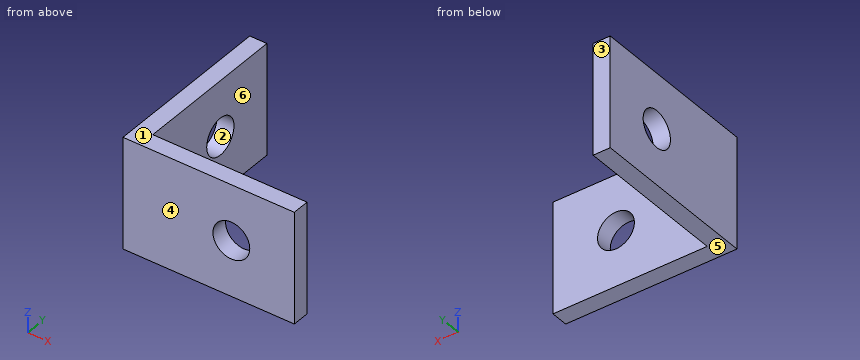
from build123d import *

# Parameters (mm, degrees)
BOSS_EXTRUDE1_DEPTH = 13
SKETCH2_R           = 2.15
CUT_EXTRUDE1_DEPTH  = 21
SKETCH3_R           = 2.15
CUT_EXTRUDE2_DEPTH  = 21


with BuildPart() as part:
    # Sketch1 → Boss-Extrude1 (new body)
    with BuildSketch(Plane.XY):
        Polygon((0, 20), (0, 0), (20, 0), (20, 2), (2, 2), (2, 20), align=None)
    extrude(amount=BOSS_EXTRUDE1_DEPTH)

    # Sketch2 → Cut-Extrude1 (cut, through all)
    with BuildSketch(Plane.ZY):
        with Locations((6.5, 12.65)):
            Circle(SKETCH2_R)
    extrude(amount=-CUT_EXTRUDE1_DEPTH, mode=Mode.SUBTRACT)

    # Sketch3 → Cut-Extrude2 (cut, through all)
    with BuildSketch(Plane.XZ):
        with Locations((12.65, 6.5)):
            Circle(SKETCH3_R)
    extrude(amount=-CUT_EXTRUDE2_DEPTH, mode=Mode.SUBTRACT)


solid = part.part
The model under review builds one solid part; all positions refer to its coordinate system, in mm. Face numbers are marked on the shaded views. A direction names the side the tool comes from. Coordinates: 2 decimals unless noted, no trailing zeros. Write each loop counter-clockwise with the first axis right and the second up, starting at its lowest first coordinate (ties: lowest second). Pieces come first, ordered by that corner, then holes. Notation, with made-up numbers: (10, -15.75) -> (55, -15.75) arc R20 cw to (55, -8.75) -> close; hole circle Ø8 at (80, 16.25). An arc over 180 degrees is marked (long way). Answer in a Markdown table with one row per item.
1. Clearance check with flat-ended pins moving along their axes: pin 1 Ø10 at (x, y) = (8, 13.5) entering from +Z; pin 2 Ø6.5 at (x, z) = (10, 9) entering from +Y; pin 3 Ø8 at (x, y) = (14.5, 5.5) entering from -Z. State where each tip first meets the part, or that it passes through.
Answers below:
| item | result |
|---|---|
| pin 1 | passes through |
| pin 2 | stops at y = 2 |
| pin 3 | stops at z = 0 |
2. We need section B-B, the plane z = 6.5. State the section outline as (x, y) points, and give its area (3 significant figures).
Answers below:
| item | result |
|---|---|
| outline | (0, 0) -> (10.5, 0) -> (10.5, 2) -> (2, 2) -> (2, 10.5) -> (0, 10.5) -> close; (0, 14.8) -> (2, 14.8) -> (2, 20) -> (0, 20) -> close; (14.8, 0) -> (20, 0) -> (20, 2) -> (14.8, 2) -> close |
| area | 58.8 mm^2 |
3. Wall thickness on probe 1 along Y at (x, z) = (0.45, 6.5); probe 2 along Z at (x, y) = (12.65, 1); probe 3 along Y at (x, z) = (7.5, 10.5): over which ranges is each line inside the solid? List them lowest first. Write a range as [from, to].
Answers below:
| item | result |
|---|---|
| probe 1 | y = [0, 10.5], [14.8, 20] |
| probe 2 | z = [0, 4.35], [8.65, 13] |
| probe 3 | y = [0, 2] |
4. We need section D-D, the plane x = 1.5. State the section outline as (y, z) points, and give its area (3 significant figures).
Answers below:
| item | result |
|---|---|
| outline | (0, 0) -> (20, 0) -> (20, 13) -> (0, 13) -> close; hole circle Ø4.3 at (12.65, 6.5) |
| area | 245 mm^2 |
5. We need section A-A, the plane x = 12.65. State the section outline as (y, z) points, and give its area (3 significant figures).
Answers below:
| item | result |
|---|---|
| outline | (0, 0) -> (2, 0) -> (2, 4.35) -> (0, 4.35) -> close; (0, 8.65) -> (2, 8.65) -> (2, 13) -> (0, 13) -> close |
| area | 17.4 mm^2 |
6. For the marked faces 5 and 6, list the 3-axis set-ups (+Z, -Z, +X, -X, +Y, -Y) from which the entire face can be reached by the end or side of a thin tool; tool diameter is ignored.
Answers below:
| item | result |
|---|---|
| face 5 | -Z, +X, -X, +Y, -Y |
| face 6 | +Z, -Z, +X, +Y |
7. Draft analysis for pull direction Y (two halves, no side actions). For the marked faces 1, 2, 3 and 4, state which applies: +Y half, -Y half, draft (parallel to the pull), parting line (faces both ways), or undercut.
Answers below:
| item | result |
|---|---|
| face 1 | draft |
| face 2 | undercut |
| face 3 | +Y half |
| face 4 | -Y half |
